For this review, take the finished solid that the model builds, in its own axes (mm). A direction names the side the tool comes from. Round coordinates to 2 decimals unless told otherwise and drop trailing zeros. Order: outer loops, then holes, each group sorted by start corner. A loop starts at its lowest first (then second) coordinate and runs counter-clockwise, first axis right, second up. Notation, with made-up numbers: M 17.25,47 L 65.25,47 A29 ccw 65.25,85 Z; hole C 18.25,50 d10. An arc over 180 degrees is marked long. Put each result on its own line as item: value.
from build123d import *

# Parameters (mm, degrees)
F0_R     = 63.5
F0_R_2   = 57.15
F1_DEPTH = 140
F2_R     = 57.15
F3_DEPTH = 172.72
F4_DEPTH = 150
F5_R     = 1.27
F6_DEPTH = 140.001


with BuildPart() as f1:
    # F0 (on Top) → F1 (new body)
    with BuildSketch(Plane.XY):
        Circle(F0_R)
        Circle(F0_R_2, mode=Mode.SUBTRACT)
        Circle(F0_R_2)
    extrude(amount=F1_DEPTH)

    # F2 (on Top) → F3 (join)
    with BuildSketch(Plane.XY):
        Circle(F2_R)
    extrude(amount=F3_DEPTH)

    # F4 (cut): faces of the model
    f4_faces = [f1.faces().sort_by_distance(p)[0] for p in [
        (0, 0, 172.72),
        (0, 0, 0),
    ]]
    extrude(f4_faces, amount=-F4_DEPTH, dir=(0, 0, 1), mode=Mode.SUBTRACT)

    # F5 (on Top) → F6 (cut, through all)
    with BuildSketch(Plane.XY):
        Circle(F5_R)
    extrude(amount=F6_DEPTH, mode=Mode.SUBTRACT)


solid = f1.part
(1) To check wall thickness, follow L1, parallel to Y at x = 0, z = 13; L2, parallel to Y at x = 0, z = 109; L3, parallel to Z at x = 21, y = -14. State the ranges of each line that lie inside material, in increasing order.
A:
L1: y = -63.5 to -1.27, 1.27 to 63.5
L2: y = -63.5 to -57.15, 57.15 to 63.5
L3: z = 0 to 22.72
(2) Add section B-B on y = -8. Give the boundary of the cut face in (x, z).
A:
outline: M -62.99,0 L 62.99,0 L 62.99,140 L 56.59,140 L 56.59,22.72 L -56.59,22.72 L -56.59,140 L -62.99,140 Z
(3) Add section D-D on z = 99.5. Give the boundary of the cut face in (x, y).
A:
outline: C 0,0 d127; hole C 0,0 d114.3
(4) Insertion check: pin 1 Ø8 at (y, z) = (23.5, 126) entering from -X; pin 2 Ø1 at (y, z) = (-50, 70.5) entering from +X; pin 3 Ø2 at (y, z) = (31, 104) entering from +X. Each pin has a flat end and moves straight along its axis. Give the tip position at first contact, or say it passes through.
A:
pin 1: stops at x = -60.43
pin 2: stops at x = 39.77
pin 3: stops at x = 55.97
(5) Add section A-A on z = 9. Give the boundary of the cut face in (x, y), then the cut area to 3 significant figures.
A:
outline: C 0,0 d127; hole C 0,0 d2.54
area: 12,700 mm2
(6) For faces 1 (the face through (-13.77, -61.99, 69.02)), 2 (the face through (-57.095, 2.513, 82.181)), list the 3-axis set-ups (+Z, -Z, +X, -X, +Y, -Y) from which the entire face can be reached by the end or side of a thin tool; tool diameter is ignored.
A:
face 1: +Z, -Z
face 2: +Z
(7) Add section C-C on x = -38. Give the boundary of the cut face in (y, z), then the cut area to 3 significant figures.
A:
outline: M -50.87,0 L 50.87,0 L 50.87,140 L 42.69,140 L 42.69,22.72 L -42.69,22.72 L -42.69,140 L -50.87,140 Z
area: 4,230 mm2
